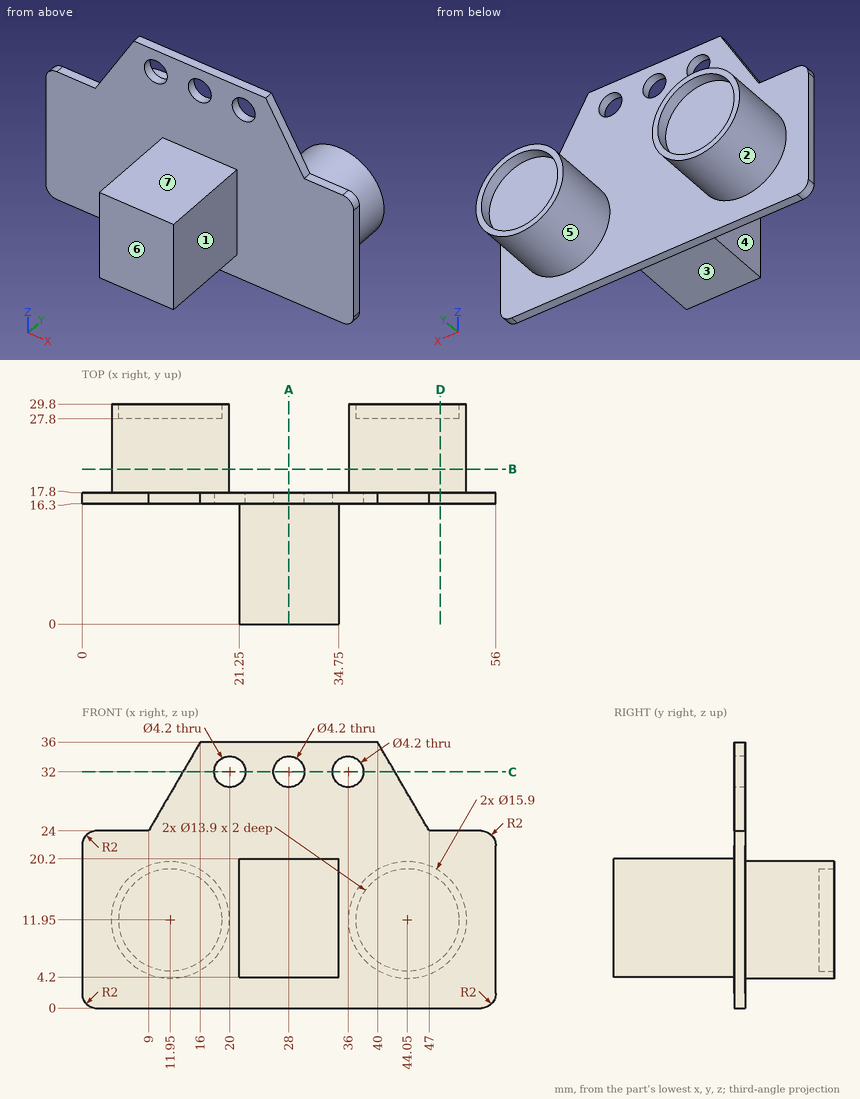
Answer from the drawing. Dimensions are ordinates in mm from the lowest x, y and z of the part. A direction names the side the tool comes from. Coordinates: 2 decimals unless noted, no trailing zeros. Order: outer loops, then holes, each group sorted by start corner. A loop starts at its lowest first (then second) coordinate and runs counter-clockwise, first axis right, second up. Notation, with made-up numbers: (-22.5, 78) -> (13.5, 78) arc R32 ccw to (13.5, 104) -> close; hole circle Ø6 at (-29, -37.75). An arc over 180 degrees is marked (long way). Answer as a JSON object with one key per item and string values.
1) A cutting plane is placed at D-D, the plane x = 48.5. Determine the outline of the cut face in (y, z).
Model answer:
{"outline": "(16.3, 0) -> (17.8, 0) -> (17.8, 5.36) -> (29.8, 5.36) -> (29.8, 6.61) -> (27.8, 6.61) -> (27.8, 17.29) -> (29.8, 17.29) -> (29.8, 18.54) -> (17.8, 18.54) -> (17.8, 24) -> (16.3, 24) -> close"}
2) A tool of negligible diameter and unlimited length cuts with its end or side. For the marked faces 4, 5, 6 and 7, from which of +Z, -Z, +X, -X, +Y, -Y can it reach the whole face along a straight path? Write none if from no direction.
Model answer:
{"face 4": "+Z, -Z, -X, -Y", "face 5": "+Y", "face 6": "+Z, -Z, +X, -X, -Y", "face 7": "+Z, +X, -X, -Y"}
3) Consider line 1 along X through (y, z) = (17.4, 32); line 2 along Y through (x, z) = (54, 23); line 3 along Z through (x, y) = (20, 17.45). Determine where each line is inside the solid, lowest interval first. Write a range as from..to.
Model answer:
{"line 1": "x = 13.67..17.9, 22.1..25.9, 30.1..33.9, 38.1..42.33", "line 2": "y = 16.3..17.8", "line 3": "z = 0..29.9, 34.1..36"}
4) Each of these flat-tipped pins is pushed along its axis until it touches: pin 1 (16 mm diameter, centred on x = 44.05, z = 11.95, fed in from -Y); pin 2 (1.5 mm diameter, centred on y = 21, z = 10, fed in from -X); pin 3 (8 mm diameter, centred on y = 5.5, z = 16, fed in from +X). Where does it stop, or does it pass through?
Model answer:
{"pin 1": "stops at y = 16.3", "pin 2": "stops at x = 4.09", "pin 3": "stops at x = 34.75"}
5) A cutting plane is placed at B-B, the plane y = 21. Determine the outline of the cut face in (x, z), plus the area to 3 significant figures.
Model answer:
{"outline": "circle Ø15.9 at (11.95, 11.95); circle Ø15.9 at (44.05, 11.95)", "area": "397 mm²"}
6) A cutting plane is placed at A-A, the plane x = 28. Determine the outline of the cut face in (y, z).
Model answer:
{"outline": "(0, 4.2) -> (16.3, 4.2) -> (16.3, 0) -> (17.8, 0) -> (17.8, 29.9) -> (16.3, 29.9) -> (16.3, 20.2) -> (0, 20.2) -> close; (16.3, 34.1) -> (17.8, 34.1) -> (17.8, 36) -> (16.3, 36) -> close"}
7) The mould has two halves that part along X. Classify the marked faces 1, 2 and 3: released by +X, released by -X, zero draft, split by the parting line, or undercut.
Model answer:
{"face 1": "released by +X", "face 2": "undercut", "face 3": "zero draft"}
8) A cutting plane is placed at C-C, the plane z = 32. Determine the outline of the cut face in (x, y).
Model answer:
{"outline": "(13.67, 16.3) -> (17.9, 16.3) -> (17.9, 17.8) -> (13.67, 17.8) -> close; (22.1, 16.3) -> (25.9, 16.3) -> (25.9, 17.8) -> (22.1, 17.8) -> close; (30.1, 16.3) -> (33.9, 16.3) -> (33.9, 17.8) -> (30.1, 17.8) -> close; (38.1, 16.3) -> (42.33, 16.3) -> (42.33, 17.8) -> (38.1, 17.8) -> close"}
